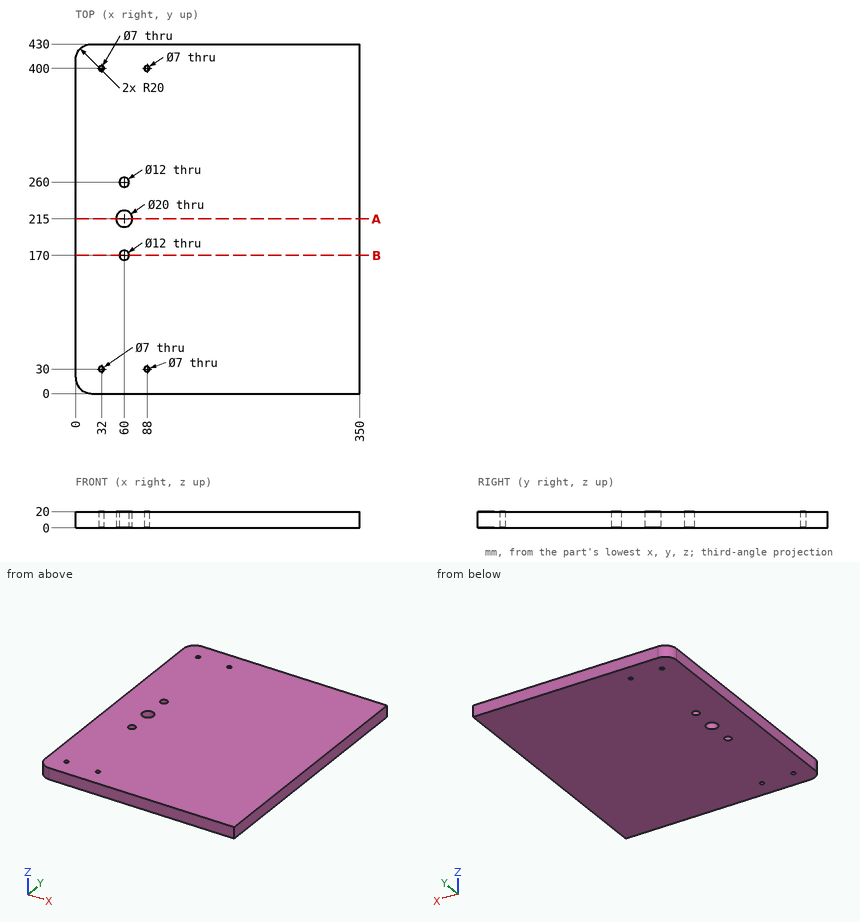
Verification items for this drawing (mm, ordinates from the low corner). Coordinates: 2 decimals unless noted, no trailing zeros. Order: outer loops, then holes, each group sorted by start corner. A loop starts at its lowest first (then second) coordinate and runs counter-clockwise, first axis right, second up. Notation, with made-up numbers: (53, -9.75) - (69, -9.75) arc R21 cw to (69, 1.25) - close; hole circle Ø10 at (77.25, 11). An arc over 180 degrees is marked (long way). Answer in a Markdown table with one row per item. Add a question column.
1. Gauge pin test, flat end, axial feed: pin 1 Ø4 at (x, y) = (32, 30) entering from +Z. Record the tip position at first contact, or that the pin passes through.
2. Section check B-B (y = 170). Enter the section's corners in (x, z).
3. Section check A-A (y = 215). Enter the section's corners in (x, z), plus the area to 3 significant figures.
4. Material ranges on L1, parallel to X at y = 400, z = 14.5; L2, parallel to Y at x = 60, z = 7.25; L3, parallel to X at y = 260, z = 8, recorded low to high. Write a range as [from, to].
Data:
| question | item | result |
|---|---|---|
| 1 | pin 1 | passes through |
| 2 | outline | (0, 0) - (54, 0) - (54, 20) - (0, 20) - close; (66, 0) - (350, 0) - (350, 20) - (66, 20) - close |
| 3 | outline | (0, 0) - (50, 0) - (50, 20) - (0, 20) - close; (70, 0) - (350, 0) - (350, 20) - (70, 20) - close |
| 3 | area | 6,600 mm² |
| 4 | L1 | x = [0, 28.5], [35.5, 84.5], [91.5, 350] |
| 4 | L2 | y = [0, 164], [176, 205], [225, 254], [266, 430] |
| 4 | L3 | x = [0, 54], [66, 350] |
